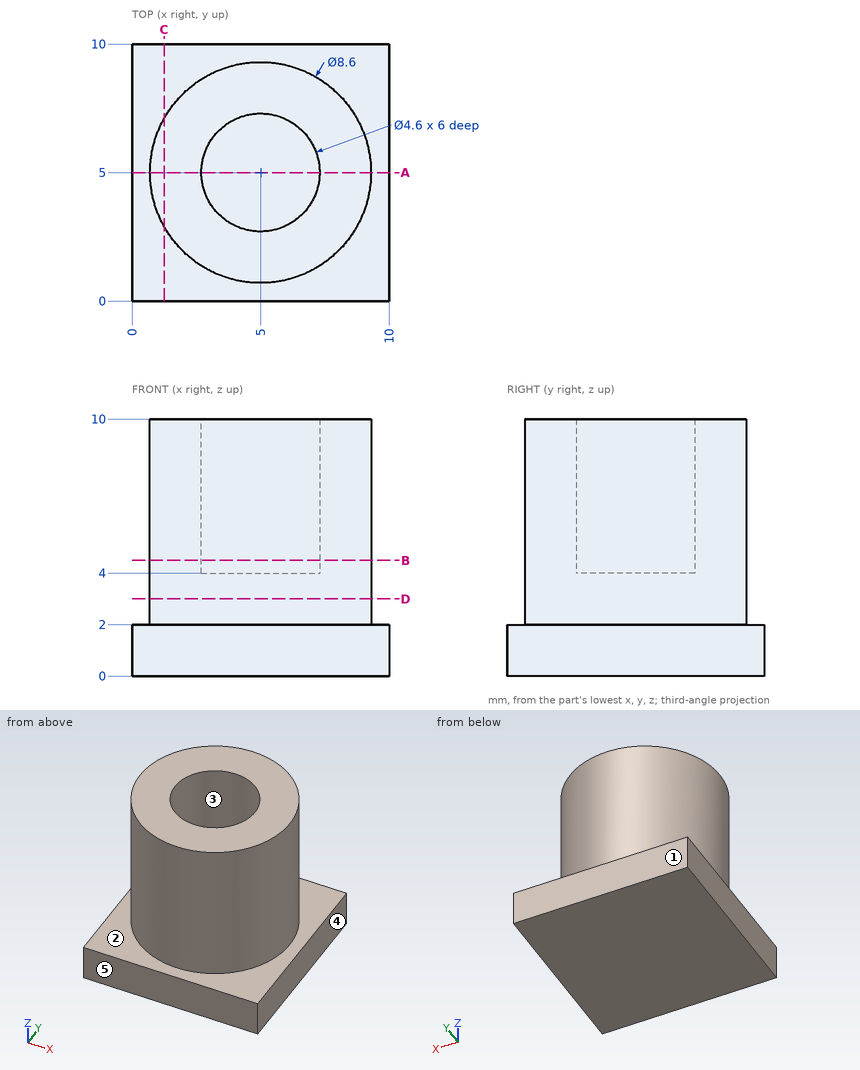
For this review, use the dimensioned drawing (mm, ordinates from the lowest corner) and the shaded views. A direction names the side the tool comes from. Round coordinates to 2 decimals unless told otherwise and drop trailing zeros. Order: outer loops, then holes, each group sorted by start corner. A loop starts at its lowest first (then second) coordinate and runs counter-clockwise, first axis right, second up. Notation, with made-up numbers: (40, 49.5) -> (48, 49.5) arc R21 cw to (48, 83.5) -> close; hole circle Ø9 at (58.5, 51). An arc over 180 degrees is marked (long way). Put each result on its own line as item: value.
Q1. Add section B-B on z = 4.5. Write out the cut boundary in (x, y), plus the area to 3 significant figures.
Check result:
outline: circle Ø8.6 at (5, 5); hole circle Ø4.6 at (5, 5)
area: 41.5 mm2
Q2. Machinability: for the marked faces 1 and 2, which of the approach directions +Z, -Z, +X, -X, +Y, -Y give a long, thin tool a straight path to every point of the face, cutting with its end or side? Answer none if there is none.
Check result:
face 1: +Z, -Z, +X, -X, +Y
face 2: +Z
Q3. Add section C-C on x = 1.25. Write out the cut boundary in (y, z), plus the area to 3 significant figures.
Check result:
outline: (0, 0) -> (10, 0) -> (10, 2) -> (7.1, 2) -> (7.1, 10) -> (2.9, 10) -> (2.9, 2) -> (0, 2) -> close
area: 53.7 mm2
Q4. For probe 1 along Y at (x, z) = (5, 5.6); probe 2 along Z at (x, y) = (9, 9); probe 3 along Y at (x, z) = (6.5, 9.75), list the stretches that pass through material, from the lowest coordinate up. Write a range as [from, to].
Check result:
probe 1: [0.7, 2.7], [7.3, 9.3]
probe 2: [0, 2]
probe 3: [0.97, 3.26], [6.74, 9.03]
Q5. Insertion check: pin 1 Ø1.4 at (x, y) = (4, 6) entering from +Z; pin 2 Ø1.5 at (y, z) = (8, 7) entering from -X; pin 3 Ø3 at (y, z) = (7.5, 4.5) entering from -X. Each pin has a flat end and moves straight along its axis. Give the tip position at first contact, or say it passes through.
Check result:
pin 1: z = 4
pin 2: x = 1.34
pin 3: x = 0.82
Q6. Mouldability with a two-part tool opening along X and no side actions: class the marked faces 3, 4 and 5 as pulls with the +X half, pulls with the -X half, needs draft (parallel to the pull), parting line crosses it, or undercut.
Check result:
face 3: undercut
face 4: pulls with the +X half
face 5: needs draft
Q7. Add section D-D on z = 3. Write out the cut boundary in (x, y).
Check result:
outline: circle Ø8.6 at (5, 5)
Q8. Add section A-A on y = 5. Write out the cut boundary in (x, z), plus the area to 3 significant figures.
Check result:
outline: (0, 0) -> (10, 0) -> (10, 2) -> (9.3, 2) -> (9.3, 10) -> (7.3, 10) -> (7.3, 4) -> (2.7, 4) -> (2.7, 10) -> (0.7, 10) -> (0.7, 2) -> (0, 2) -> close
area: 61.2 mm2
